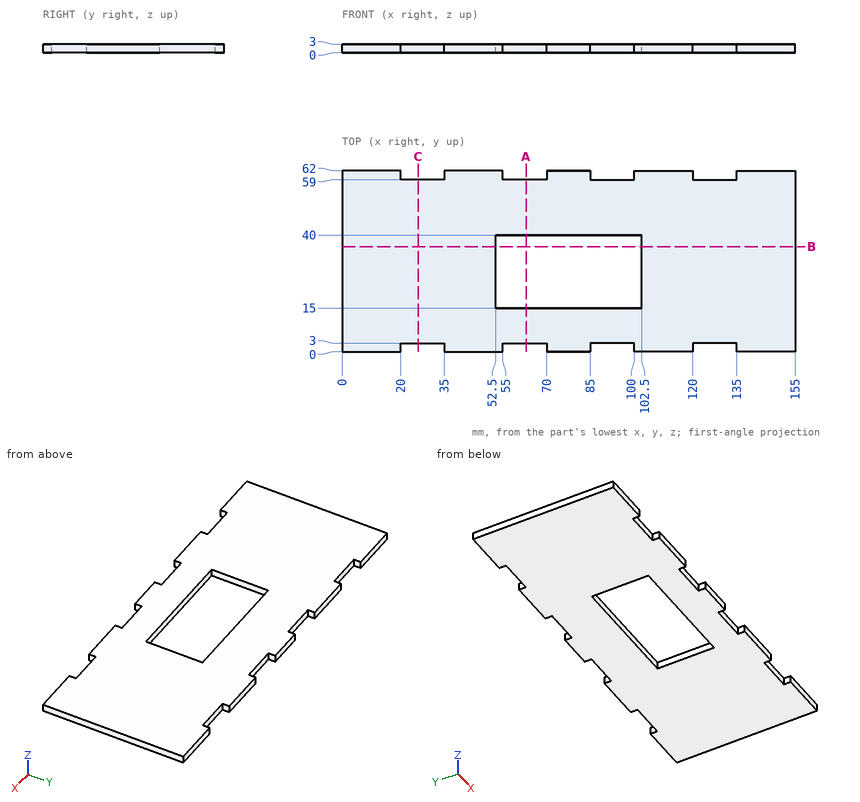
Here's the drawing with two shaded views (mm, measured from the low corner). I have some questions. Coordinates: 2 decimals unless noted, no trailing zeros. Loops run counter-clockwise (first coordinate to the right, second up) from the corner with the lowest first, then second, coordinate; pieces in that order, holes last.
Item 1: Suppose I cut it at B-B (y = 36). Please give me the cut outline in (x, z), then the cut area to 3 significant figures.
Answers below:
outline: (0, 0) - (52.5, 0) - (52.5, 3) - (0, 3) - close; (102.5, 0) - (155, 0) - (155, 3) - (102.5, 3) - close
area: 315 mm2
Item 2: Suppose I cut it at C-C (x = 26). Please give me the cut outline in (y, z), then the cut area to 3 significant figures.
Answers below:
outline: (3, 0) - (59, 0) - (59, 3) - (3, 3) - close
area: 168 mm2
Item 3: Please list where these lines run through material, in increasing order: L1, parallel to Y at x = 84, z = 1.5; L2, parallel to Y at x = 67.5, z = 1.1; L3, parallel to X at y = 30.5, z = 2.8.
Answers below:
L1: y = 0 to 15, 40 to 62
L2: y = 3 to 15, 40 to 59
L3: x = 0 to 52.5, 102.5 to 155
Item 4: Suppose I cut it at A-A (x = 63). Please give me the cut outline in (y, z).
Answers below:
outline: (3, 0) - (15, 0) - (15, 3) - (3, 3) - close; (40, 0) - (59, 0) - (59, 3) - (40, 3) - close
Item 5: I'm going to push flat-ended pins straight in: pin 1 (1.5 mm diameter, centred on x = 131, z = 2, fed in from -Y); pin 2 (1.5 mm diameter, centred on x = 90.5, z = 2, fed in from +Y). Where does each tip first touch, or does it pass through?
Answers below:
pin 1: stops at y = 3
pin 2: stops at y = 59
